Geometry check sheet. Reference: the model listing, model coordinates, mm. Face numbers are marked on the shaded views. Coordinates: 2 decimals unless noted, no trailing zeros. Write each loop counter-clockwise with the first axis right and the second up, starting at its lowest first coordinate (ties: lowest second). Pieces come first, ordered by that corner, then holes. Notation, with made-up numbers: (43.25, 0) -> (90.25, 0) arc R13 cw to (90.25, 5) -> close; hole circle Ø1 at (-10, -30). An arc over 180 degrees is marked (long way). Answer in a Markdown table with one row per item. Add a question column.
1. Cross-section at A-A on x = 0. Record the cut outline in (y, z), and give its area (3 significant figures).
2. Scan lines: L1, parallel to X at y = -37.5, z = 0; L2, parallel to X at y = -20, z = -5.5; L3, parallel to Z at x = 8.5, y = -38. Record each from-to range of solid material in increasing order. Write a range as from..to.
3. Mould release check, pull along Z, two halves, no side actions. Record for the marked faces 1, 2 and 3: pulls with the +Z half, pulls with the -Z half, needs draft (parallel to the pull), parting line crosses it, or undercut.
4. Cross-section at D-D on y = -14.5. Record the cut outline in (x, z).
5. Depth check by flat-ended pin: P1, Ø8, axis at x = 18, z = -17, coming from the -Y side; P2, Ø5, axis at x = -12, z = 3, coming from the +Y side; P3, Ø8, axis at x = -19, z = -3.5, coming from the -Y side. Enter the tip coordinate at first touch or a pass-through.
6. Cross-section at B-B on z = 0. Record the cut outline in (x, y), and give its area (3 significant figures).
7. Cross-section at C-C on y = -23. Record the cut outline in (x, z), and give its area (3 significant figures).
```python
from build123d import *

# Parameters (mm, degrees)
SKETCH4_W = 0.9
SKETCH4_H = 0.8


with BuildPart() as part:
    # Sketch3 → Revolve3 (revolve)
    with BuildSketch(Plane.XY, mode=Mode.PRIVATE) as revolve3_sk:
        Polygon((-11, -44), (-10.2, -44), (-10.2, -21.754642132), (-23.575538943, -2), (-29, -2), (-29, -2.8), (-28, -2.8), (-28, -3.8), (-21.291666667, -6.8), (-11, -22), align=None)
    revolve(revolve3_sk.sketch.rotate(Axis((0, 0, 0), (0, 1, 0)), 270), axis=Axis((0, 0, 0), (0, 1, 0)))

    # Sketch4 → Cut-Revolve1 (revolve, cut)
    with BuildSketch(Plane.XY, mode=Mode.PRIVATE) as cut_revolve1_sk:
        with Locations((-28.55, -2.4)):
            Rectangle(SKETCH4_W, SKETCH4_H)
    revolve(cut_revolve1_sk.sketch.rotate(Axis((0, 0, 0), (0, -1, 0)), 270), axis=Axis((0, 0, 0), (0, -1, 0)), mode=Mode.SUBTRACT)

    # Sketch5 → Cut-Revolve2 (revolve, cut)
    with BuildSketch(Plane.XY, mode=Mode.PRIVATE) as cut_revolve2_sk:
        Polygon((-21.291666667, -6.8), (-28, -3.8), (-28, -2.8), align=None)
    revolve(cut_revolve2_sk.sketch.rotate(Axis((0, 0, 0), (0, -1, 0)), 270), axis=Axis((0, 0, 0), (0, -1, 0)), mode=Mode.SUBTRACT)


solid = part.part
```
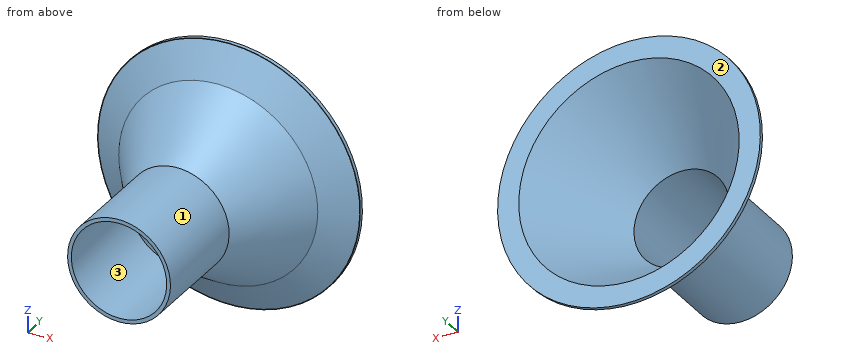
Results found:
| question | item | result |
|---|---|---|
| 1 | outline | (-44, -11) -> (-22, -11) -> (-6.8, -21.29) -> (-2.8, -28) -> (-2.8, -28.1) -> (-2, -28.1) -> (-2, -23.58) -> (-21.75, -10.2) -> (-44, -10.2) -> close; (-44, 10.2) -> (-21.75, 10.2) -> (-2, 23.58) -> (-2, 28.1) -> (-2.8, 28.1) -> (-2.8, 28) -> (-6.8, 21.29) -> (-22, 11) -> (-44, 11) -> close |
| 1 | area | 95.9 mm^2 |
| 2 | L1 | x = -11..-10.2, 10.2..11 |
| 2 | L2 | x = -11.06..-9.97, 9.97..11.06 |
| 2 | L3 | z = -6.98..-5.64, 5.64..6.98 |
| 3 | face 1 | parting line crosses it |
| 3 | face 2 | needs draft |
| 3 | face 3 | undercut |
| 4 | outline | circle Ø32.16 at (0, 0); hole circle Ø30.22 at (0, 0) |
| 5 | P1 | stops at y = -7.59 |
| 5 | P2 | stops at y = -14.86 |
| 5 | P3 | stops at y = -15.62 |
| 6 | outline | (-28.1, -2.8) -> (-28, -2.8) -> (-21.29, -6.8) -> (-11, -22) -> (-11, -44) -> (-10.2, -44) -> (-10.2, -21.75) -> (-23.58, -2) -> (-28.1, -2) -> close; (10.2, -44) -> (11, -44) -> (11, -22) -> (21.29, -6.8) -> (28, -2.8) -> (28.1, -2.8) -> (28.1, -2) -> (23.58, -2) -> (10.2, -21.75) -> close |
| 6 | area | 95.9 mm^2 |
| 7 | outline | circle Ø22 at (0, 0); hole circle Ø20.4 at (0, 0) |
| 7 | area | 53.3 mm^2 |
